The model under review builds one solid part; all positions refer to its coordinate system, in mm. Face numbers are marked on the shaded views. A direction names the side the tool comes from. Round coordinates to 2 decimals unless told otherwise and drop trailing zeros. Write each loop counter-clockwise with the first axis right and the second up, starting at its lowest first coordinate (ties: lowest second). Pieces come first, ordered by that corner, then holes. Notation, with made-up numbers: (68.25, 6.25) -> (112.25, 6.25) arc R15 ccw to (112.25, 32.25) -> close; hole circle Ø1 at (2, 26.5). An arc over 180 degrees is marked (long way). Use CSV: the item, a comma, the result in double quotes. Start each with the question number.
1) Take a section at B-B, the plane x = 0. Give the boundary of the cut face in (y, z).
2) Machinability: for the marked faces 1, 2 and 3, which of the approach directions +Z, -Z, +X, -X, +Y, -Y give a long, thin tool a straight path to every point of the face, cutting with its end or side? Answer none if there is none.
3) For pin 1 Ø4 at (x, z) = (-7.5, 135) entering from -Y; pin 2 Ø4 at (y, z) = (-3.5, 123) entering from -X; pin 3 Ø6 at (x, y) = (-4, 9.5) entering from -Z; pin 4 Ø5.5 at (x, z) = (0, 116.2) entering from -Y, all flat-tipped, find the tip position at first contact; note any pin that passes through.
4) Take a section at D-D, the plane z = 13. Give the boundary of the cut face in (x, y).
5) Wall thickness on probe 1 along Z at (x, y) = (0, 7); probe 2 along Z at (x, y) = (0, 3); probe 3 along X at (y, z) = (0.75, 141.2): over which ranges is each line inside the solid? List them lowest first. Write a range as [from, to].
6) Take a section at C-C, the plane z = 125.5. Give the boundary of the cut face in (x, y).
7) Take a section at A-A, the plane y = 0. Give the boundary of the cut face in (x, z), then the cut area to 3 significant figures.
from build123d import *

# Parameters (mm, degrees)
SKETCH1_R           = 6
BOSS_EXTRUDE1_DEPTH = 15
SKETCH2_R           = 12.5
BOSS_EXTRUDE2_DEPTH = 7
SKETCH3_R           = 12
BOSS_EXTRUDE3_DEPTH = 136.7
SKETCH4_R           = 4.5
CUT_EXTRUDE1_DEPTH  = 160.681526796
LPATTERN1_COUNT     = 2
LPATTERN1_PITCH     = 25


with BuildPart() as part:
    # Sketch1 → Boss-Extrude1 (new body)
    with BuildSketch(Plane.XY):
        Circle(SKETCH1_R)
    extrude(amount=BOSS_EXTRUDE1_DEPTH)

    # Sketch2 → Boss-Extrude2 (add)
    with BuildSketch(Plane.XY.offset(15)):
        Circle(SKETCH2_R)
    extrude(amount=BOSS_EXTRUDE2_DEPTH)

    # Sketch3 → Boss-Extrude3 (add)
    with BuildSketch(Plane.XY.offset(22)):
        Circle(SKETCH3_R)
    extrude(amount=BOSS_EXTRUDE3_DEPTH)

    # Sketch4 → Cut-Extrude1 (cut, symmetric)
    with BuildSketch(Plane(origin=(0, 0, 0), x_dir=(1, 0, 0), z_dir=(0, 1, 0))):
        with Locations(Location((0, -141.2, 0), (0, 0, 270))):
            Circle(SKETCH4_R)
    cut_extrude1 = extrude(amount=CUT_EXTRUDE1_DEPTH, both=True, mode=Mode.SUBTRACT)

    # LPattern1: Cut-Extrude1 ×2
    with Locations(*[(0, 0, -i * LPATTERN1_PITCH) for i in range(1, LPATTERN1_COUNT)]):
        add(cut_extrude1, mode=Mode.SUBTRACT)


solid = part.part
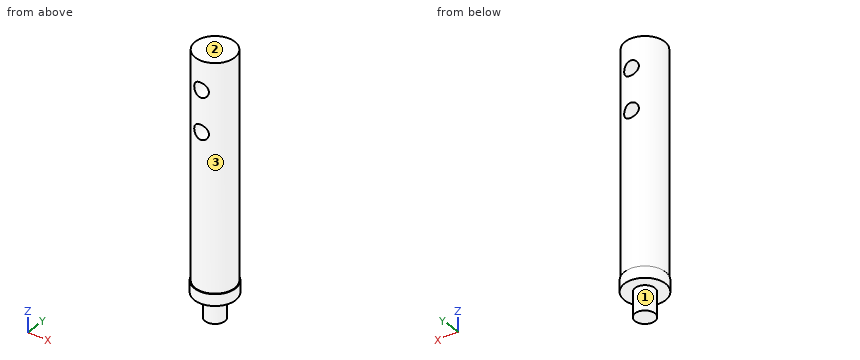
Values found:
1,outline,"(-12.5, 15) -> (-6, 15) -> (-6, 0) -> (6, 0) -> (6, 15) -> (12.5, 15) -> (12.5, 22) -> (12, 22) -> (12, 111.7) -> (-12, 111.7) -> (-12, 22) -> (-12.5, 22) -> close; (-12, 120.7) -> (12, 120.7) -> (12, 136.7) -> (-12, 136.7) -> close; (-12, 145.7) -> (12, 145.7) -> (12, 158.7) -> (-12, 158.7) -> close"
2,face 1,"-Z"
2,face 2,"+Z, +X, -X, +Y, -Y"
2,face 3,"+Z"
3,pin 1,"y = -10.67"
3,pin 2,"x = -11.91"
3,pin 3,"z = 15"
3,pin 4,"through"
4,outline,"circle Ø12 at (0, 0)"
5,probe 1,"[15, 111.7], [120.7, 136.7], [145.7, 158.7]"
5,probe 2,"[0, 111.7], [120.7, 136.7], [145.7, 158.7]"
5,probe 3,"[-11.98, -4.5], [4.5, 11.98]"
6,outline,"circle Ø24 at (0, 0)"
7,outline,"(-12.5, 15) -> (-6, 15) -> (-6, 0) -> (6, 0) -> (6, 15) -> (12.5, 15) -> (12.5, 22) -> (12, 22) -> (12, 158.7) -> (-12, 158.7) -> (-12, 22) -> (-12.5, 22) -> close; hole circle Ø9 at (0, 116.2); hole circle Ø9 at (0, 141.2)"
7,area,"3,510 mm²"
